Check sheet for the modelled part. Datum: model origin and axes. Units: mm. Face numbers are marked on the shaded views. A direction names the side the tool comes from. Coordinates: 2 decimals unless noted, no trailing zeros. Write each question's results on one line, items separated by ' | '.
from build123d import *

# Parameters (mm, degrees)
F0_R     = 1.5
F0_R_2   = 2
F1_DEPTH = 2
F2_SIZE  = 1.99999
F3_R     = 4
F3_R_2   = 2
F4_DEPTH = 6


# Not quite as in the source:
# - a fillet or chamfer is up to 0.001 mm smaller than in the source, because OpenCascade refuses the exact size


with BuildPart() as f1:
    # F0 (on Front) → F1 (new body)
    with BuildSketch(Plane.XZ):
        with BuildLine():
            Line((-10.6066017178, -3.5355339059), (-3.5355339059, -10.6066017178))
            ThreePointArc((-3.5355339059, -10.6066017178), (0, -12.0710678119), (3.5355339059, -10.6066017178))
            Line((3.5355339059, -10.6066017178), (10.6066017178, -3.5355339059))
            ThreePointArc((10.6066017178, -3.5355339059), (12.0710678119, 0), (10.6066017178, 3.5355339059))
            Line((10.6066017178, 3.5355339059), (3.5355339059, 10.6066017178))
            ThreePointArc((3.5355339059, 10.6066017178), (0, 12.0710678119), (-3.5355339059, 10.6066017178))
            Line((-3.5355339059, 10.6066017178), (-10.6066017178, 3.5355339059))
            ThreePointArc((-10.6066017178, 3.5355339059), (-12.0710678119, 0), (-10.6066017178, -3.5355339059))
        make_face()
        with Locations((-7, 0)):
            Circle(F0_R, mode=Mode.SUBTRACT)
        with Locations((0, -7)):
            Circle(F0_R, mode=Mode.SUBTRACT)
        Circle(F0_R_2, mode=Mode.SUBTRACT)
        with Locations((7, 0)):
            Circle(F0_R, mode=Mode.SUBTRACT)
        with Locations((0, 7)):
            Circle(F0_R, mode=Mode.SUBTRACT)
    extrude(amount=F1_DEPTH)

    # F2 (size 2 in the source; OpenCascade refuses exactly that, so slightly less here)
    f2_edges = [f1.edges().sort_by_distance(p)[0] for p in [
        (5.5, -2, 0),
        (-1.5, -2, -7),
        (-8.5, -2, 0),
        (-1.5, -2, 7),
    ]]
    chamfer(f2_edges, length=F2_SIZE)

    # F3 (on face) → F4 (join)
    with BuildSketch(Plane(origin=(0, 0, 0), x_dir=(-1, 0, 0), z_dir=(0, 1, 0))):
        Circle(F3_R)
        Circle(F3_R_2, mode=Mode.SUBTRACT)
    extrude(amount=F4_DEPTH)


solid = f1.part
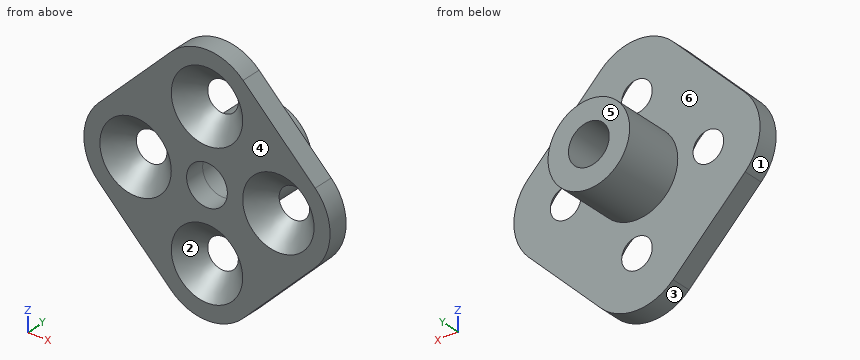
1. Go/stop test with flat-tipped pins: pin 1 (1 mm diameter, centred on x = 5, z = 6, fed in from +Y); pin 2 (3.5 mm diameter, centred on x = 0, z = 7, fed in from -Y); pin 3 (1.8 mm diameter, centred on x = -7, z = 0, fed in from -Y). Record where each tip stops, or that it passes through.
Values follow:
pin 1: stops at y = 0 | pin 2: stops at y = -0.25 | pin 3: passes through
2. Draft check along Z on the marked faces 1, 2, 3 and 4. Enter one of: pulls with the +Z half, pulls with the -Z half, needs draft (parallel to the pull), parting line crosses it, or undercut.
Values follow:
face 1: parting line crosses it | face 2: undercut | face 3: pulls with the -Z half | face 4: needs draft
3. Access from +Z, -Z, +X, -X, +Y, -Y to the whole of each face (thin tool, end or side, straight path). Record for the marked faces 5 and 6.
Values follow:
face 5: +Z, -Z, +X, -X, +Y | face 6: +Y
4. Sectioned sample at A-A (z = 0). Give the number of separate pieces and of enclosed holes in the cut face, then the cut area to 3 significant figures.
Values follow:
separate pieces: 4 | enclosed holes: 0 | area: 44.3 mm^2
5. Material ranges on L1, parallel to Z at x = 0, y = -0.5; L2, parallel to Z at x = 0, y = 1.5; L3, parallel to X at y = -0.7, z = 0, recorded low to high. Write a range as [from, to].
Values follow:
L1: z = [-12.07, -9], [-5, -2], [2, 5], [9, 12.07] | L2: z = [-4, -2], [2, 4] | L3: x = [-12.07, -9.2], [-4.8, -2], [2, 4.8], [9.2, 12.07]
